Geometry check sheet. Reference: drawing and pictorial views, mm from the part's lowest x, y, z. A direction names the side the tool comes from. Give positions to 0.01 mm unless a question says otherwise; leave off trailing zeros. Loops run counter-clockwise (first coordinate to the right, second up) from the corner with the lowest first, then second, coordinate; pieces in that order, holes last. Notation, with made-up numbers: (44.25, 6.5) -> (95.25, 6.5) arc R30 ccw to (95.25, 43.5) -> close; hole circle Ø6 at (36.25, 73.5). An arc over 180 degrees is marked (long way). Write each question's results on one line, items separated by ' | '. Start each with the question number.
1. Gauge pin test, flat end, axial feed: pin 1 Ø1.5 at (y, z) = (1.5, 21.5) entering from -X. Record the tip position at first contact, or that the pin passes through.
2. Cross-section at D-D on z = 47.5. Record the boundary of the cut face in (x, y), and give its area (3 significant figures).
3. Material ranges on L1, parallel to Z at x = 12.5, y = 2.75; L2, parallel to X at y = 5, z = 30; L3, parallel to Z at x = 21, y = 1.5, recorded low to high. Write a range as from..to.
4. Cross-section at A-A on y = 3. Record the boundary of the cut face in (x, z).
5. Cross-section at C-C on x = 24. Record the boundary of the cut face in (y, z).
6. Cross-section at B-B on z = 62. Record the boundary of the cut face in (x, y), and give its area (3 significant figures).
7. Tool access check on the marked faces 1, 2 and 3. Record the directions out of +Z, -Z, +X, -X, +Y, -Y that give a thin tool (end or side, any length) a straight path to the whole face; none if there is none.
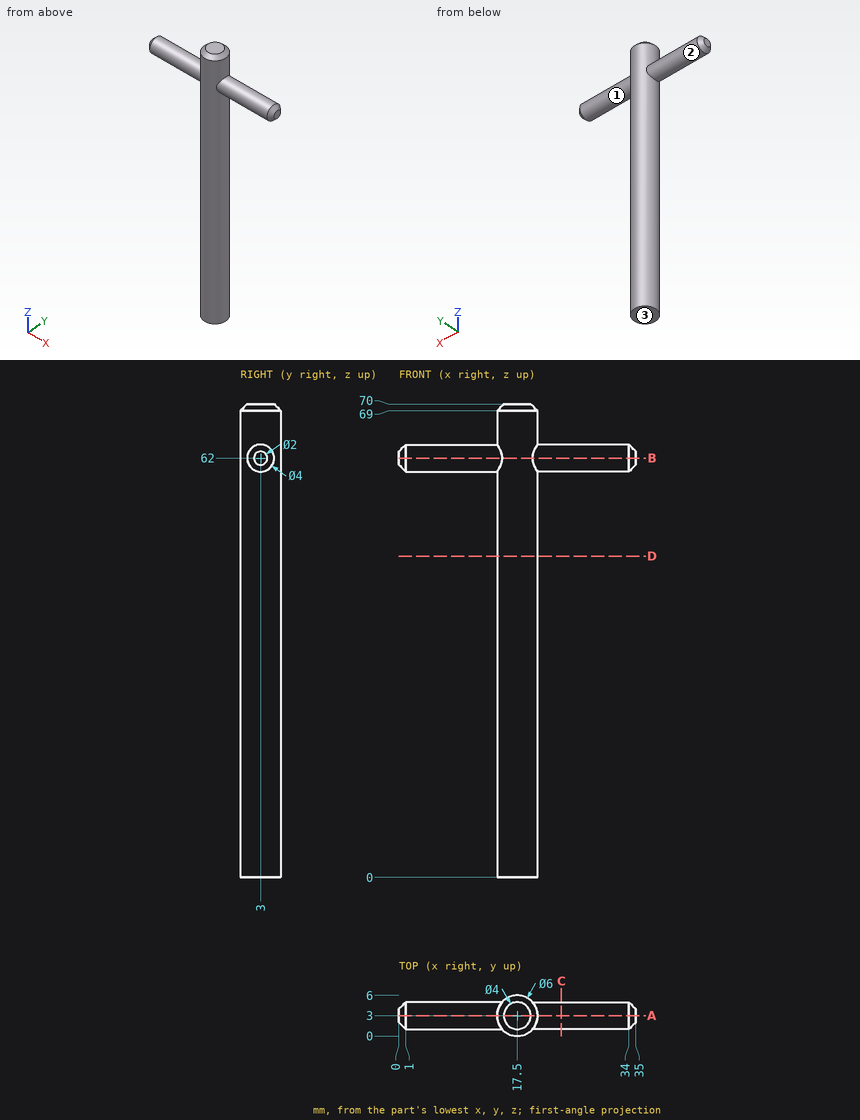
Geometry says:
1) pin 1: x = 14.6
2) outline: circle Ø6 at (17.5, 3) | area: 28.3 mm^2
3) L1: 60.02..63.98 | L2: 15.26..19.74 | L3: 60.68..63.32
4) outline: (0, 61) -> (1, 60) -> (14.5, 60) -> (14.5, 0) -> (20.5, 0) -> (20.5, 60) -> (34, 60) -> (35, 61) -> (35, 63) -> (34, 64) -> (20.5, 64) -> (20.5, 69) -> (19.5, 70) -> (15.5, 70) -> (14.5, 69) -> (14.5, 64) -> (1, 64) -> (0, 63) -> close
5) outline: circle Ø4 at (3, 62)
6) outline: (0, 2) -> (1, 1) -> (15.26, 1) arc R3 ccw to (19.74, 1) -> (34, 1) -> (35, 2) -> (35, 4) -> (34, 5) -> (19.74, 5) arc R3 ccw to (15.26, 5) -> (1, 5) -> (0, 4) -> close | area: 144 mm^2
7) face 1: +X | face 2: -X | face 3: -Z, +X, -X, +Y, -Y
